from build123d import *

# Parameters (mm, degrees)
SKETCH3_R           = 100
BOSS_EXTRUDE1_DEPTH = 22.5
CHAMFER1_SIZE       = 10
CUT_EXTRUDE1_DEPTH  = 25.25
CIRPATTERN1_COUNT   = 6
SKETCH5_R           = 15
CUT_EXTRUDE2_DEPTH  = 22.5


with BuildPart() as part:
    # Sketch3 → Boss-Extrude1 (new body)
    with BuildSketch(Plane(origin=(0, 0, 0), x_dir=(1, 0, 0), z_dir=(0, 1, 0))):
        with Locations(Location((0, 0, 0), (0, 0, 90))):
            Circle(SKETCH3_R)
    extrude(amount=BOSS_EXTRUDE1_DEPTH)

    # Chamfer1
    chamfer1_edges = [part.edges().sort_by_distance(p)[0] for p in [
        (0, 22.5, 100),
    ]]
    chamfer(chamfer1_edges, length=CHAMFER1_SIZE)

    # Sketch4 → Cut-Extrude1 (cut, symmetric)
    with BuildSketch(Plane.XY):
        Polygon((-75.630877335, 0), (-72.480463966, 9.69597536), (-71.909830056, 9.510565163), (-75, 0), align=None)
    cut_extrude1 = extrude(amount=CUT_EXTRUDE1_DEPTH, both=True, mode=Mode.SUBTRACT)

    # CirPattern1: Cut-Extrude1 ×6 about axis
    cirpattern1_axis = Axis((0, 0, 0), (0, 1, 0))
    for i in range(1, CIRPATTERN1_COUNT):
        add(cut_extrude1.rotate(cirpattern1_axis, i * 360 / CIRPATTERN1_COUNT), mode=Mode.SUBTRACT)

    # Sketch5 → Cut-Extrude2 (cut)
    with BuildSketch(Plane(origin=(0, 22.5, 0), x_dir=(1, 0, 0), z_dir=(0, 1, 0))):
        with Locations(Location((0, 0, 0), (0, 0, 270))):
            Circle(SKETCH5_R)
    extrude(amount=-CUT_EXTRUDE2_DEPTH, mode=Mode.SUBTRACT)


solid = part.part
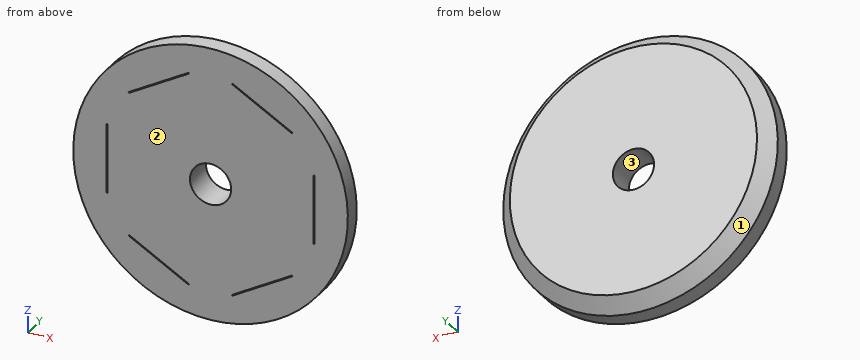
For this review, take the finished solid that the model builds, in its own axes (mm). Face numbers are marked on the shaded views. Round coordinates to 2 decimals unless told otherwise and drop trailing zeros. Write each loop counter-clockwise with the first axis right and the second up, starting at its lowest first coordinate (ties: lowest second). Pieces come first, ordered by that corner, then holes. Notation, with made-up numbers: (53.25, -20.75) -> (77.25, -20.75) arc R8 ccw to (77.25, -5.75) -> close; hole circle Ø1 at (53.25, 52). An arc over 180 degrees is marked (long way). Use CSV: the item, a comma, the result in double quotes.
(1) Consider section C-C, the plane y = 19.25. Give the boundary of the cut face in (x, z), plus the area to 3 significant figures.
Computed values:
outline,"circle Ø186.5 at (0, 0); hole circle Ø30 at (0, 0)"
area,"26,600 mm²"
(2) Consider section B-B, the plane z = 0. Give the boundary of the cut face in (x, y).
Computed values:
outline,"(-100, 0) -> (-75.63, 0) -> (-72.48, 9.7) -> (-71.91, 9.51) -> (-75, 0) -> (-15, 0) -> (-15, 22.5) -> (-90, 22.5) -> (-100, 12.5) -> close; (15, 0) -> (75, 0) -> (71.91, 9.51) -> (72.48, 9.7) -> (75.63, 0) -> (100, 0) -> (100, 12.5) -> (90, 22.5) -> (15, 22.5) -> close"
(3) Consider section D-D, the plane y = 4.5. Give the boundary of the cut face in (x, z).
Computed values:
outline,"circle Ø200 at (0, 0); hole (-74.17, -25.25) -> (-73.54, -25.25) -> (-73.54, 25.25) -> (-74.17, 25.25) -> close; hole (-58.95, -51.61) -> (-15.22, -76.86) -> (-14.9, -76.31) -> (-58.64, -51.06) -> close; hole (-58.95, 51.61) -> (-58.64, 51.06) -> (-14.9, 76.31) -> (-15.22, 76.86) -> close; hole circle Ø30 at (0, 0); hole (14.9, -76.31) -> (15.22, -76.86) -> (58.95, -51.61) -> (58.64, -51.06) -> close; hole (14.9, 76.31) -> (58.64, 51.06) -> (58.95, 51.61) -> (15.22, 76.86) -> close; hole (73.54, -25.25) -> (74.17, -25.25) -> (74.17, 25.25) -> (73.54, 25.25) -> close"
(4) Clearance check with flat-ended pins moving along their axes: P1, Ø3, axis at x = -73, y = 2.5, coming from the -Z side; P2, Ø12, axis at x = 71.5, y = 12, coming from the +Z side; P3, Ø4, axis at x = 73.5, y = 4.5, coming from the +Z side. State where each tip first meets the part, or that it passes through.
Computed values:
P1,"z = -69.91"
P2,"z = 75.56"
P3,"z = 69.91"
(5) To check wall thickness, follow L1, parallel to X at y = 11.75, z = 0; L2, parallel to Z at x = 18, y = 8.75; L3, parallel to Z at x = -58, y = 2.25. State the ranges of each line that lie inside material, in increasing order. Write a range as [from, to].
Computed values:
L1,"[-100, -15], [15, 100]"
L2,"[-98.37, -73.66], [-72.93, 72.93], [73.66, 98.37]"
L3,"[-81.46, -53], [-52.27, 52.27], [53, 81.46]"
(6) Consider section A-A, the plane x = 0. Give the boundary of the cut face in (y, z).
Computed values:
outline,"(0, -100) -> (12.5, -100) -> (22.5, -90) -> (22.5, -15) -> (0, -15) -> close; (0, 15) -> (22.5, 15) -> (22.5, 90) -> (12.5, 100) -> (0, 100) -> close"
(7) Draft analysis for pull direction Z (two halves, no side actions). For the marked faces 1, 2 and 3, state which applies: +Z half, -Z half, draft (parallel to the pull), parting line (faces both ways), or undercut.
Computed values:
face 1,"parting line"
face 2,"draft"
face 3,"undercut"
